```python
from build123d import *

# Parameters (mm, degrees)
SKETCH1_R             = 3
SKETCH1_R_2           = 1
BOSS_EXTRUDE1_DEPTH   = 7.2
BOSS_EXTRUDE1_2_DEPTH = 7.2
BOSS_EXTRUDE1_3_DEPTH = 7.2
BOSS_EXTRUDE1_4_DEPTH = 7.2
BOSS_EXTRUDE2_START   = -3
SKETCH2_R             = 1.5
BOSS_EXTRUDE2_DEPTH   = 3
FILLET1_R             = 10


with BuildPart() as part:
    # Sketch1 → Boss-Extrude1 (new body)
    with BuildSketch(Plane(origin=(49.162852783, 0, 0), x_dir=(0, 0, -1), z_dir=(1, 0, 0))):
        with Locations(Location((0.658959109, 5.919497669, 0), (0, 0, 270))):
            Circle(SKETCH1_R)
        with Locations(Location((0.658959109, 5.919497669, 0), (0, 0, 270))):
            Circle(SKETCH1_R_2, mode=Mode.SUBTRACT)
    extrude(amount=BOSS_EXTRUDE1_DEPTH)



with BuildPart() as body_2:
    # Sketch1 → Boss-Extrude1 2 (new body)
    with BuildSketch(Plane(origin=(49.162852783, 0, 0), x_dir=(0, 0, -1), z_dir=(1, 0, 0))):
        with Locations(Location((0.658959109, -14.080502331, 0), (0, 0, 270))):
            Circle(SKETCH1_R)
        with Locations(Location((0.658959109, -14.080502331, 0), (0, 0, 270))):
            Circle(SKETCH1_R_2, mode=Mode.SUBTRACT)
    extrude(amount=BOSS_EXTRUDE1_2_DEPTH)


with BuildPart() as body_3:
    # Sketch1 → Boss-Extrude1 3 (new body)
    with BuildSketch(Plane(origin=(49.162852783, 0, 0), x_dir=(0, 0, -1), z_dir=(1, 0, 0))):
        with Locations(Location((16.658959109, -14.080502331, 0), (0, 0, 270))):
            Circle(SKETCH1_R)
        with Locations(Location((16.658959109, -14.080502331, 0), (0, 0, 270))):
            Circle(SKETCH1_R_2, mode=Mode.SUBTRACT)
    extrude(amount=BOSS_EXTRUDE1_3_DEPTH)


with BuildPart() as body_4:
    # Sketch1 → Boss-Extrude1 4 (new body)
    with BuildSketch(Plane(origin=(49.162852783, 0, 0), x_dir=(0, 0, -1), z_dir=(1, 0, 0))):
        with Locations(Location((16.658959109, 5.919497669, 0), (0, 0, 270))):
            Circle(SKETCH1_R)
        with Locations(Location((16.658959109, 5.919497669, 0), (0, 0, 270))):
            Circle(SKETCH1_R_2, mode=Mode.SUBTRACT)
    extrude(amount=BOSS_EXTRUDE1_4_DEPTH)


with BuildPart() as part_1:
    add(part.part)

    add(body_2.part)  # Boss-Extrude2 merges body 2

    add(body_3.part)  # Boss-Extrude2 merges body 3

    add(body_4.part)  # Boss-Extrude2 merges body 4
    # Sketch2 → Boss-Extrude2 (add)
    with BuildSketch(Plane(origin=(56.362852783, 0, 0), x_dir=(0, 0, -1), z_dir=(1, 0, 0)).offset(BOSS_EXTRUDE2_START)):
        with BuildLine():
            Line((-0.336368494, 6.016053158), (-10.432923983, -4.080502331))
            Line((-10.432923983, -4.080502331), (-0.336368494, -14.17705782))
            ThreePointArc((-0.336368494, -14.17705782), (1.366065891, -13.373395549), (0.562403621, -15.075829934))
            Line((0.562403621, -15.075829934), (8.658959109, -23.172385423))
            Line((8.658959109, -23.172385423), (16.755514598, -15.075829934))
            ThreePointArc((16.755514598, -15.075829934), (15.951852328, -13.373395549), (17.654286713, -14.17705782))
            Line((17.654286713, -14.17705782), (27.750842202, -4.080502331))
            Line((27.750842202, -4.080502331), (17.654286713, 6.016053158))
            ThreePointArc((17.654286713, 6.016053158), (15.951852328, 5.212390888), (16.755514598, 6.914825272))
            Line((16.755514598, 6.914825272), (8.658959109, 15.011380761))
            Line((8.658959109, 15.011380761), (0.562403621, 6.914825272))
            ThreePointArc((0.562403621, 6.914825272), (1.366065891, 5.212390888), (-0.336368494, 6.016053158))
        make_face()
        with Locations((-3.361856171, -4.080502331)):
            Circle(SKETCH2_R, mode=Mode.SUBTRACT)
        with BuildLine():
            ThreePointArc((-2.745060132, -7.525725494), (0.138143829, -4.080502331), (-2.745060132, -0.635279167))
            Line((-2.745060132, -0.635279167), (5.213735946, 7.323516911))
            ThreePointArc((5.213735946, 7.323516911), (8.658959109, 4.440312949), (12.104182273, 7.323516911))
            Line((12.104182273, 7.323516911), (20.062978351, -0.635279167))
            ThreePointArc((20.062978351, -0.635279167), (17.17977439, -4.080502331), (20.062978351, -7.525725494))
            Line((20.062978351, -7.525725494), (12.104182273, -15.484521572))
            ThreePointArc((12.104182273, -15.484521572), (8.658959109, -12.601317611), (5.213735946, -15.484521572))
            Line((5.213735946, -15.484521572), (-2.745060132, -7.525725494))
        make_face(mode=Mode.SUBTRACT)
        with Locations((8.658959109, -16.101317611)):
            Circle(SKETCH2_R, mode=Mode.SUBTRACT)
        with Locations((20.67977439, -4.080502331)):
            Circle(SKETCH2_R, mode=Mode.SUBTRACT)
        with Locations((8.658959109, 7.940312949)):
            Circle(SKETCH2_R, mode=Mode.SUBTRACT)
    extrude(amount=BOSS_EXTRUDE2_DEPTH)

    # Fillet1
    # the kernel refuses this fillet: 10 mm, written as the material it takes off along each edge
    with BuildSketch(Plane(origin=(30.395755029, 15.011380761, -8.658959109), x_dir=(0, -0.7071067811865511, -0.7071067811865438), z_dir=(1, 0, 0)), Plane(origin=(30.395755029, -23.172385423, -8.658959109), x_dir=(0, 0.7071067811865509, 0.707106781186544), z_dir=(1, 0, 0))) as fillet1_piece_1:
        with BuildLine():
            CenterArc((9.969337782, -9.969337782), FILLET1_R, 94.487975167, 81.024049665)
            Line((0, -9.186839102), (0, 0))
            Line((0, 0), (9.186839102, 0))
        make_face()
    extrude(amount=48.934195508, mode=Mode.SUBTRACT)
    with BuildSketch(Plane(origin=(28.362852783, -4.080502331, -27.750842202), x_dir=(-4.937700262164531e-15, -0.7071067811865436, 0.7071067811865513), z_dir=(1, 0, 0))) as fillet1_piece_2:
        with BuildLine():
            CenterArc((FILLET1_R, -FILLET1_R), FILLET1_R, 90, 90)
            Line((0, -FILLET1_R), (0, 0))
            Line((0, 0), (FILLET1_R, 0))
        make_face()
    extrude(amount=53, mode=Mode.SUBTRACT)
    with BuildSketch(Plane(origin=(28.362852783, -4.080502331, 10.432923983), x_dir=(0, -0.7071067811865515, -0.7071067811865436), z_dir=(1, 0, 0))) as fillet1_piece_3:
        with BuildLine():
            CenterArc((FILLET1_R, FILLET1_R), FILLET1_R, 180, 90)
            Line((0, FILLET1_R), (0, 0))
            Line((0, 0), (FILLET1_R, 0))
        make_face()
    extrude(amount=53, mode=Mode.SUBTRACT)


solid = part_1.part
```
Can you work these out from the model? Positions are in its coordinate system, mm. A direction names the side the tool comes from. Give positions to 0.01 mm unless a question says otherwise; leave off trailing zeros. Write each loop counter-clockwise with the first axis right and the second up, starting at its lowest first coordinate (ties: lowest second). Pieces come first, ordered by that corner, then holes. Notation, with made-up numbers: (45, 37) - (95, 37) arc R13 ccw to (95, 56) - close; hole circle Ø7 at (56.25, 6.25). An arc over 180 degrees is marked (long way). Write item = value, one per line. Start each with the question number.
1. Imagine slicing it at A-A (x = 52.75). Please give me the cut outline in (y, z), and give its area (3 significant figures).
2. For pin 1 (3.5 mm diameter, centred on y = -4.5, z = -21, fed in from -X), with a flat end and sliding along its axis, tell me the tip position at first contact or that it passes through.
3. On a 3-axis mill with a long thin cutter (end or side, diameter ignored), from which of +Z, -Z, +X, -X, +Y, -Y can I reach the whole of each face in a straight line? I mean faces 4 (the face through (54.84, -9.33, 0.94)), 5 (the face through (49.163, -14, -15)). Say none if no direction works.
4. Imagine slicing it at C-C (y = 3.5). Please give me the cut outline in (x, z), and give its area (3 significant figures).
5. Thinking about a two-plate mould opening in Z: for faces 1 (the face through (54.842, -11.854, 2.659)), 2 (the face through (54.84, -14.72, -4.45)), 3 (the face through (49.163, 4.6, -0.7)), which applies, released by +Z, released by -Z, zero draft, split by the parting line, or undercut?
6. Imagine slicing it at B-B (z = -21.25). Please give me the cut outline in (x, y), and give its area (3 significant figures).
7. Imagine slicing it at D-D (z = -11.5). Please give me the cut outline in (x, y), and give its area (3 significant figures).
8. Please list where these lines run through material, in increasing order: line 1 (Y direction, x = 52.25, z = -1); line 2 (Z direction, x = 55.75, y = -5.25); line 3 (Z direction, x = 54.5, y = 7).
Worked answers:
q1.outline = circle Ø6 at (-14.08, -16.66); circle Ø6 at (-14.08, -0.66); circle Ø6 at (5.92, -16.66); circle Ø6 at (5.92, -0.66); hole circle Ø2 at (-14.08, -16.66); hole circle Ø2 at (-14.08, -0.66); hole circle Ø2 at (5.92, -16.66); hole circle Ø2 at (5.92, -0.66)
q1.area = 101 mm2
q2.pin_1 = 53.36
q3.face_4 = +X, -X
q3.face_5 = +Z, -Z, -X, +Y, -Y
q4.outline = (49.16, -18.43) - (53.36, -18.43) - (53.36, -20.17) - (56.36, -20.17) - (56.36, -14.89) - (49.16, -14.89) - close; (49.16, -2.43) - (56.36, -2.43) - (56.36, 2.85) - (53.36, 2.85) - (53.36, 1.11) - (49.16, 1.11) - close
q4.area = 61.5 mm2
q5.face_1 = released by +Z
q5.face_2 = undercut
q5.face_3 = zero draft
q6.outline = (53.36, -10.53) - (56.36, -10.53) - (56.36, -5.47) - (53.36, -5.47) - close; (53.36, -2.69) - (56.36, -2.69) - (56.36, 2.37) - (53.36, 2.37) - close
q6.area = 30.4 mm2
q7.outline = (53.36, -18.66) - (56.36, -18.66) - (56.36, -14.06) - (53.36, -14.06) - close; (53.36, 5.9) - (56.36, 5.9) - (56.36, 10.5) - (53.36, 10.5) - close
q7.area = 27.6 mm2
q8.line_1 = -17.06 to -15.02, -13.14 to -11.1, 2.94 to 4.98, 6.86 to 8.9
q8.line_2 = -23.54 to -21.62, -19.74 to -17.38, 0.06 to 2.42, 4.3 to 6.22
q8.line_3 = -19.46 to -12.43, -12.03 to -9.83, -7.49 to -5.29, -4.89 to 2.14
